```python
from build123d import *

# Parameters (mm, degrees)
BOSS_EXTRUDE1_DEPTH       = 50.8
F_6_32_TAPPED_HOLE1_D     = 2.7051
F_6_32_TAPPED_HOLE1_DEPTH = 9.398
F_6_32_TAPPED_HOLE1_TIP   = 0.81269403
F_6_32_TAPPED_HOLE2_D     = 2.7051
F_6_32_TAPPED_HOLE2_DEPTH = 9.398
F_6_32_TAPPED_HOLE2_TIP   = 0.81269403


with BuildPart() as part:
    # Sketch1 → Boss-Extrude1 (new body)
    with BuildSketch(Plane(origin=(0, 0, 0), x_dir=(1, 0, 0), z_dir=(0, 1, 0))):
        Polygon((3.175, 1.833087105), (0, 3.666174209), (-3.175, 1.833087105), (-3.175, -1.833087105), (0, -3.666174209), (3.175, -1.833087105), align=None)
    extrude(amount=BOSS_EXTRUDE1_DEPTH)

    # #6-32 Tapped Hole1
    with Locations(Plane(origin=(0, 50.8, 0), x_dir=(-1, 0, 0), z_dir=(0, 1, 0))):
        with Locations((0.023544291, 0.002414528)):
            Hole(F_6_32_TAPPED_HOLE1_D / 2, depth=F_6_32_TAPPED_HOLE1_DEPTH)
            with Locations((0, 0, -(F_6_32_TAPPED_HOLE1_DEPTH + F_6_32_TAPPED_HOLE1_TIP / 2))):  # 118° drill point
                Cone(0, F_6_32_TAPPED_HOLE1_D / 2, F_6_32_TAPPED_HOLE1_TIP, mode=Mode.SUBTRACT)

    # #6-32 Tapped Hole2
    with Locations(Plane.XZ):
        with Locations((0.021072049, 0.073538109)):
            Hole(F_6_32_TAPPED_HOLE2_D / 2, depth=F_6_32_TAPPED_HOLE2_DEPTH)
            with Locations((0, 0, -(F_6_32_TAPPED_HOLE2_DEPTH + F_6_32_TAPPED_HOLE2_TIP / 2))):  # 118° drill point
                Cone(0, F_6_32_TAPPED_HOLE2_D / 2, F_6_32_TAPPED_HOLE2_TIP, mode=Mode.SUBTRACT)


solid = part.part
```
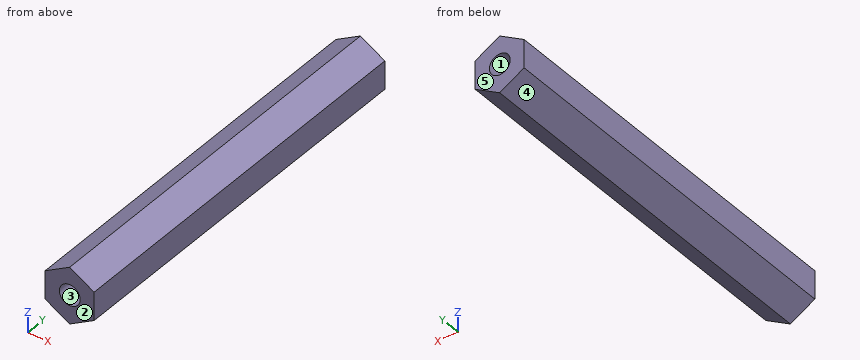
Check sheet for the modelled part. Datum: model origin and axes. Units: mm. Face numbers are marked on the shaded views. A direction names the side the tool comes from. Round coordinates to 2 decimals unless told otherwise and drop trailing zeros. Loops run counter-clockwise (first coordinate to the right, second up) from the corner with the lowest first, then second, coordinate; pieces in that order, holes last. Notation, with made-up numbers: (28, 45) - (77, 45) arc R27 ccw to (77, 64) - close; hole circle Ø1 at (-25.5, 81.25). An arc over 180 degrees is marked (long way). Answer as a JSON object with one key per item and string values. Group by question number.
Q1. Mould release check, pull along X, two halves, no side actions. Record for the marked faces 3, 4 and 5: released by +X, released by -X, zero draft, split by the parting line, or undercut.
Q2. Gauge pin test, flat ends, axial feed: P1, Ø1, axis at y = 34.5, z = 2, coming from the -X side (3 decimals); P2, Ø1.6, axis at x = -0.02, z = 0, coming from the -Y side. Record the tip position at first contact, or that the pin passes through.
Q3. Scan lines: line 1 along X through (y, z) = (2.5, 0) (3 decimals); line 2 along Z through (x, y) = (0.25, 43); line 3 along Z through (x, y) = (-1, 4.5). Record each from-to range of solid material in increasing order. Write a range as [from, to].
Q4. Sectioned sample at C-C, the plane z = 3. Enter the section's corners in (x, y).
Q5. Sectioned sample at A-A, the plane y = 27. Enter the section's corners in (x, z) (3 decimals), plus the area to 3 significant figures.
Q6. Sectioned sample at B-B, the plane y = 6.5. Enter the section's corners in (x, z) (3 decimals).
Q7. Sectioned sample at D-D, the plane x = -2.25. Enter the section's corners in (y, z), plus the area to 3 significant figures.
Q8. Set-up check for the marked faces 1 and 2: record each of +Z, -Z, +X, -X, +Y, -Y from which the full face is reachable in a straight line by a thin tool's end or side.
Solution:
{
 "1": {"face 3": "undercut", "face 4": "released by -X", "face 5": "zero draft"},
 "2": {"P1": "stops at x = -3.175", "P2": "stops at y = 9.68"},
 "3": {"line 1": "x = [-3.175, -1.329], [1.372, 3.175]", "line 2": "z = [-3.52, -1.32], [1.33, 3.52]", "line 3": "z = [-3.09, -0.81], [0.96, 3.09]"},
 "4": {"outline": "(-1.15, 0) - (1.15, 0) - (1.15, 50.8) - (-1.15, 50.8) - close"},
 "5": {"outline": "(-3.175, -1.833) - (0, -3.666) - (3.175, -1.833) - (3.175, 1.833) - (0, 3.666) - (-3.175, 1.833) - close", "area": "34.9 mm²"},
 "6": {"outline": "(-3.175, -1.833) - (0, -3.666) - (3.175, -1.833) - (3.175, 1.833) - (0, 3.666) - (-3.175, 1.833) - close; hole circle Ø2.705 at (0.021, 0.074)"},
 "7": {"outline": "(0, -2.37) - (50.8, -2.37) - (50.8, 2.37) - (0, 2.37) - close", "area": "241 mm²"},
 "8": {"face 1": "+Y", "face 2": "+Z, -Z, +X, -X, -Y"}
}
